from build123d import *

# Parameters (mm, degrees)
BOSS_EXTRUDE1_DEPTH = 70
CUT_EXTRUDE1_DEPTH  = 65
SKETCH6_W           = 80
SKETCH6_H           = 36
BOSS_EXTRUDE2_DEPTH = 12
SKETCH7_W           = 71
SKETCH7_H           = 27
CUT_EXTRUDE2_DEPTH  = 20


with BuildPart() as part:
    # Sketch1 → Boss-Extrude1 (new body)
    with BuildSketch(Plane(origin=(0, 0, 0), x_dir=(1, 0, 0), z_dir=(0, 1, 0))):
        Polygon((57.735026919, -100), (100, -57.735026919), (-100, -57.735026919), (-57.735026919, -100), (0, -115.470053838), align=None)
    extrude(amount=BOSS_EXTRUDE1_DEPTH)

    # Sketch4 → Cut-Extrude1 (cut)
    with BuildSketch(Plane(origin=(0, 70, 0), x_dir=(1, 0, 0), z_dir=(0, 1, 0))):
        Polygon((110.293672936, 0), (95.517122639, 55.146836468), (55.146836468, 95.517122639), (0, 110.293672936), (-55.146836468, 95.517122639), (-95.517122639, 55.146836468), (-110.293672936, 0), (-95.517122639, -55.146836468), (-55.146836468, -95.517122639), (0, -110.293672936), (55.146836468, -95.517122639), (95.517122639, -55.146836468), align=None)
    extrude(amount=-CUT_EXTRUDE1_DEPTH, mode=Mode.SUBTRACT)

    # Sketch6 → Boss-Extrude2 (add)
    with BuildSketch(Plane.XY.offset(104.5)):
        with Locations((0, 45)):
            Rectangle(SKETCH6_W, SKETCH6_H)
    extrude(amount=BOSS_EXTRUDE2_DEPTH)

    # Sketch7 → Cut-Extrude2 (cut)
    with BuildSketch(Plane.XY.offset(116.5)):
        with Locations((0, 45)):
            Rectangle(SKETCH7_W, SKETCH7_H)
    extrude(amount=-CUT_EXTRUDE2_DEPTH, mode=Mode.SUBTRACT)


solid = part.part
Design review of the part built by this model. Coordinates are the model's own, in mm. A direction names the side the tool comes from. Round coordinates to 2 decimals unless told otherwise and drop trailing zeros. Order: outer loops, then holes, each group sorted by start corner. A loop starts at its lowest first (then second) coordinate and runs counter-clockwise, first axis right, second up. Notation, with made-up numbers: M 60,15 L 111,15 A6 ccw 111,23 Z; hole C 12.5,-3 d6. An arc over 180 degrees is marked long. Answer as CSV lines item,"result". Start each with the question number.
1) Add section C-C (z = 88). Give the boundary of the cut face in (x, y), then the cut area to 3 significant figures.
2) For pin 1 Ø1.3 at (x, y) = (4, 30) entering from -Z; pin 2 Ø3 at (x, z) = (13, 93) entering from +Y; pin 3 Ø3 at (y, z) = (23.5, 70) entering from +X (3 decimals), all flat-tipped, find the tip position at first contact; note any pin that passes through.
3) Tool access review of faces 5 (the face through (0, 29, 104.5)), 6 (the face through (0, 27, 107)), 7 (the face through (40, 45, 111)), 8 (the face through (0, 31.5, 110)): name each direction out of +Z, -Z, +X, -X, +Y, -Y from which nothing blocks a thin tool from reaching the whole face with its end or side.
4) Add section A-A (y = 45). Give the boundary of the cut face in (x, z), then the cut area to 3 significant figures.
5) Add section D-D (x = 49). Give the boundary of the cut face in (y, z), then the cut area to 3 significant figures.
6) Wall thickness on line 1 along Y through (x, z) = (-43.5, 98); line 2 along X through (y, z) = (55.5, 112.5); line 3 along X through (y, z) = (8, 87.5): over which ranges is each line inside the solid? List them lowest first. Write a range as [from, to].
7) The part is to be moulded in two halves that separate along X. For faces 1 (the face through (34.878, 26.732, 106.124)), 2 (the face through (8, 4, 57.735)), 3 (the face through (-40, 45, 111)), 4 (the face through (-1, 5, 78)), say which applies: +X half, -X half, draft (parallel to the pull), parting line (faces both ways), or undercut.
8) Add section B-B (y = 65.5). Give the boundary of the cut face in (x, z), then the cut area to 3 significant figures.
Resolved:
1,outline,"M -69.74,0 L 69.74,0 L 69.74,70 L 62.66,70 L 62.66,5 L -62.66,5 L -62.66,70 L -69.74,70 Z"
1,area,"1,620 mm^2"
2,pin 1,"z = 104.5"
2,pin 2,"y = 5"
2,pin 3,"x = 89.235"
3,face 5,"-Z, +Y"
3,face 6,"-Z"
3,face 7,"+Z, +X, +Y, -Y"
3,face 8,"+Z, -Z"
4,outline,"M -100,57.74 L -92.93,57.74 L -55.15,95.52 L -35.5,100.78 L -35.5,116.5 L -40,116.5 L -40,104.75 L -57.74,100 Z; M 35.5,100.78 L 55.15,95.52 L 92.93,57.74 L 100,57.74 L 57.74,100 L 40,104.75 L 40,116.5 L 35.5,116.5 Z"
4,area,"883 mm^2"
5,outline,"M 0,57.74 L 5,57.74 L 5,97.16 L 70,97.16 L 70,102.34 L 0,102.34 Z"
5,area,"559 mm^2"
6,line 1,"[0, 5]"
6,line 2,"[-40, -35.5], [35.5, 40]"
6,line 3,"[-70.24, -63.16], [63.16, 70.24]"
7,face 1,"+X half"
7,face 2,"draft"
7,face 3,"-X half"
7,face 4,"undercut"
8,outline,"M -100,57.74 L -92.93,57.74 L -55.15,95.52 L 0,110.29 L 55.15,95.52 L 92.93,57.74 L 100,57.74 L 57.74,100 L 0,115.47 L -57.74,100 Z"
8,area,"1,150 mm^2"
